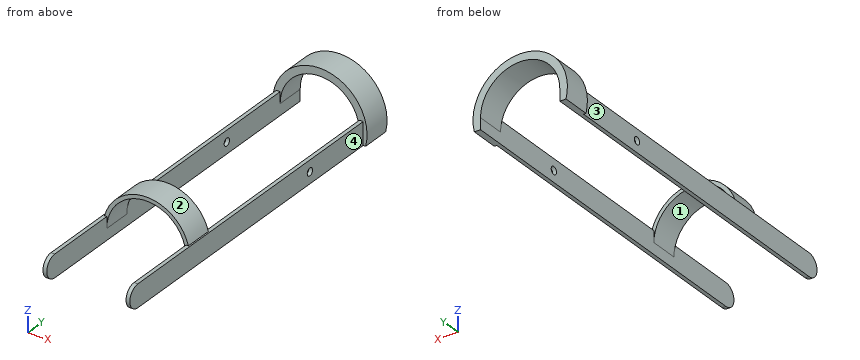
```python
from build123d import *

# Parameters (mm, degrees)
EXTRUDE_1_DEPTH     = 30
SKETCH_2_W          = 4
SKETCH_2_H          = 24
EXTRUDE_2_DEPTH     = 120
CUT_EXTRUDE_1_DEPTH = 137.674796506
SKETCH_4_W          = 4
SKETCH_4_H          = 24
EXTRUDE_3_DEPTH     = 260
EXTRUDE_START       = -30
EXTRUDE_4_DEPTH     = 30
SKETCH_6_R          = 4
CUT_EXTRUDE_2_DEPTH = 310.541596559


with BuildPart() as part:
    # 草图1 → 凸台-拉伸1 (new body)
    with BuildSketch(Plane(origin=(0, 0, 0), x_dir=(1, 0, 0), z_dir=(0, 1, 0))):
        with BuildLine():
            Line((-46, 0), (-46, 12))
            Line((-46, 12), (-42, 12))
            Line((-42, 12), (-42, 0))
            ThreePointArc((-42, 0), (0, -42), (42, 0))
            Line((42, 0), (42, 12))
            Line((42, 12), (46, 12))
            Line((46, 12), (46, 0))
            ThreePointArc((46, 0), (0, -46), (-46, 0))
        make_face()
    extrude(amount=EXTRUDE_1_DEPTH)

    # 草图2 → 凸台-拉伸2 (add)
    with BuildSketch(Plane(origin=(0, 30, 0), x_dir=(1, 0, 0), z_dir=(0, 1, 0))):
        with Locations((-44, 0)):
            Rectangle(SKETCH_2_W, SKETCH_2_H)
        with Locations((44, 0)):
            Rectangle(SKETCH_2_W, SKETCH_2_H)
    extrude(amount=-EXTRUDE_2_DEPTH)

    # 草图3 → 切除-拉伸1 (cut, through all)
    with BuildSketch(Plane(origin=(46, 0, 0), x_dir=(0, 0, -1), z_dir=(1, 0, 0))):
        with BuildLine():
            Line((-12, -78), (-12, -98.506149354))
            Line((-12, -98.506149354), (12, -98.506149354))
            Line((12, -98.506149354), (12, -78))
            ThreePointArc((12, -78), (0, -90), (-12, -78))
        make_face()
    extrude(amount=-CUT_EXTRUDE_1_DEPTH, mode=Mode.SUBTRACT)

    # 草图4 → 凸台-拉伸3 (add)
    with BuildSketch(Plane(origin=(0, 30, 0), x_dir=(1, 0, 0), z_dir=(0, 1, 0))):
        with Locations((44, 0)):
            Rectangle(SKETCH_4_W, SKETCH_4_H)
        with Locations((-44, 0)):
            Rectangle(SKETCH_4_W, SKETCH_4_H)
    extrude(amount=EXTRUDE_3_DEPTH)

    # 草图5 → 凸台-拉伸4 (add)
    with BuildSketch(Plane(origin=(0, 290, 0), x_dir=(1, 0, 0), z_dir=(0, 1, 0)).offset(EXTRUDE_START)):
        with BuildLine():
            Line((-48.538644398, 12), (-42, 12))
            Line((-42, 12), (-42, 0))
            ThreePointArc((-42, 0), (0, -42), (42, 0))
            Line((42, 0), (42, 12))
            Line((42, 12), (48.538644398, 12))
            ThreePointArc((48.538644398, 12), (0, -50), (-48.538644398, 12))
        make_face()
    extrude(amount=EXTRUDE_4_DEPTH)

    # 草图6 → 切除-拉伸2 (cut, through all)
    with BuildSketch(Plane(origin=(46, 0, 0), x_dir=(0, 0, -1), z_dir=(1, 0, 0))):
        with Locations((0, 180)):
            Circle(SKETCH_6_R)
    extrude(amount=-CUT_EXTRUDE_2_DEPTH, mode=Mode.SUBTRACT)


solid = part.part
```
The listing builds one solid part. Answer for the finished solid, in the listing's coordinates (mm). Face numbers are marked on the shaded views. Coordinates: 2 decimals unless noted, no trailing zeros. Loops run counter-clockwise (first coordinate to the right, second up) from the corner with the lowest first, then second, coordinate; pieces in that order, holes last. Notation, with made-up numbers: (8, 68.25) -> (21, 68.25) arc R22 ccw to (21, 77.25) -> close; hole circle Ø1 at (59.25, 46). An arc over 180 degrees is marked (long way). Use one line per item in the form item = value. Start each with the question number.
Item 1: The part is cut by section D-D on x = -32.5. Determine the outline of the cut face in (y, z), then the cut area to 3 significant figures.
Item 2: The part is cut by section A-A on x = 0. Determine the outline of the cut face in (y, z), then the cut area to 3 significant figures.
Item 3: The mould has two halves that part along X. Classify the marked faces 1, 2, 3 and 4: released by +X, released by -X, zero draft, split by the parting line, or undercut.
Item 4: The part is cut by section C-C on y = 180. Determine the outline of the cut face in (x, z), then the cut area to 3 significant figures.
Item 5: The part is cut by section B-B on z = 20. Determine the outline of the cut face in (x, y), then the cut area to 3 significant figures.
Item 6: Consider L1, parallel to Y at x = -0.5, z = 44.5; L2, parallel to X at y = 244, z = -4.5; L3, parallel to Y at x = -44.25, z = 0. Determine where each line is inside the solid, lowest interval first. Write a range as [from, to].
Item 7: Flat-ended cylindrical pins translate along their axes: pin 1 Ø2 at (x, y) = (-44, 170.5) entering from +Z; pin 2 Ø5 at (y, z) = (125.5, -2.5) entering from +X; pin 3 Ø13 at (y, z) = (180, 0) entering from -X. Find the tip coordinate at first contact, or state that the pin passes through.
Answer key:
q1.outline = (0, 26.6) -> (30, 26.6) -> (30, 32.55) -> (0, 32.55) -> close; (260, 26.6) -> (290, 26.6) -> (290, 38) -> (260, 38) -> close
q1.area = 520 mm2
q2.outline = (0, 42) -> (30, 42) -> (30, 46) -> (0, 46) -> close; (260, 42) -> (290, 42) -> (290, 50) -> (260, 50) -> close
q2.area = 360 mm2
q3.face_1 = undercut
q3.face_2 = split by the parting line
q3.face_3 = released by -X
q3.face_4 = released by +X
q4.outline = (-46, -12) -> (-42, -12) -> (-42, -4) -> (-46, -4) -> close; (-46, 4) -> (-42, 4) -> (-42, 12) -> (-46, 12) -> close; (42, -12) -> (46, -12) -> (46, -4) -> (42, -4) -> close; (42, 4) -> (46, 4) -> (46, 12) -> (42, 12) -> close
q4.area = 128 mm2
q5.outline = (-45.83, 260) -> (-36.93, 260) -> (-36.93, 290) -> (-45.83, 290) -> close; (-41.42, 0) -> (-36.93, 0) -> (-36.93, 30) -> (-41.42, 30) -> close; (36.93, 0) -> (41.42, 0) -> (41.42, 30) -> (36.93, 30) -> close; (36.93, 260) -> (45.83, 260) -> (45.83, 290) -> (36.93, 290) -> close
q5.area = 803 mm2
q6.L1 = [0, 30], [260, 290]
q6.L2 = [-46, -42], [42, 46]
q6.L3 = [-90, 176], [184, 290]
q7.pin_1 = 12
q7.pin_2 = 46
q7.pin_3 = -46
